Work out the finished part from the listing and answer in its coordinate system (mm). Coordinates: 2 decimals unless noted, no trailing zeros. One line per item, written item: value.
```python
from build123d import *

# Parameters (mm, degrees)
SZKIC1_R                    = 3.4
DODANIE_WYCI_GNI_CIE1_DEPTH = 820


with BuildPart() as part:
    # Szkic1 → Dodanie-wyciągnięcie1 (new body)
    with BuildSketch(Plane.XY):
        with BuildLine():
            Line((-40, -19), (-40, 19))
            ThreePointArc((-40, 19), (-39.707106781, 19.707106781), (-39, 20))
            Line((-39, 20), (-24, 20))
            Line((-24, 20), (-24, 15.5))
            Line((-24, 15.5), (-26.471381771, 15.5))
            Line((-26.471381771, 15.5), (-26.471381771, 17.75))
            ThreePointArc((-26.471381771, 17.75), (-28.062372029, 17.090990258), (-28.721381771, 15.5))
            ThreePointArc((-28.721381771, 15.5), (-27.448087912, 10.962546258), (-24, 7.75))
            Line((-24, 7.75), (-16, 7.75))
            ThreePointArc((-16, 7.75), (-12.551912088, 10.962546258), (-11.278618229, 15.5))
            ThreePointArc((-11.278618229, 15.5), (-11.937627971, 17.090990258), (-13.528618229, 17.75))
            Line((-13.528618229, 17.75), (-13.528618229, 15.5))
            Line((-13.528618229, 15.5), (-16, 15.5))
            Line((-16, 15.5), (-16, 20))
            Line((-16, 20), (13.528618229, 20))
            Line((13.528618229, 20), (16, 20))
            Line((16, 20), (16, 15.5))
            Line((16, 15.5), (13.528618229, 15.5))
            Line((13.528618229, 15.5), (13.528618229, 17.75))
            ThreePointArc((13.528618229, 17.75), (11.937627971, 17.090990258), (11.278618229, 15.5))
            ThreePointArc((11.278618229, 15.5), (12.551912088, 10.962546258), (16, 7.75))
            Line((16, 7.75), (24, 7.75))
            ThreePointArc((24, 7.75), (27.448087912, 10.962546258), (28.721381771, 15.5))
            ThreePointArc((28.721381771, 15.5), (28.062372029, 17.090990258), (26.471381771, 17.75))
            Line((26.471381771, 17.75), (26.471381771, 15.5))
            Line((26.471381771, 15.5), (24, 15.5))
            Line((24, 15.5), (24, 20))
            Line((24, 20), (39, 20))
            ThreePointArc((39, 20), (39.707106781, 19.707106781), (40, 19))
            Line((40, 19), (40, 4))
            Line((40, 4), (35.5, 4))
            Line((35.5, 4), (35.5, 6.471381771))
            Line((35.5, 6.471381771), (37.75, 6.471381771))
            ThreePointArc((37.75, 6.471381771), (37.090990258, 8.062372029), (35.5, 8.721381771))
            ThreePointArc((35.5, 8.721381771), (30.962546258, 7.448087912), (27.75, 4))
            Line((27.75, 4), (27.75, -4))
            ThreePointArc((27.75, -4), (30.962546258, -7.448087912), (35.5, -8.721381771))
            ThreePointArc((35.5, -8.721381771), (37.090990258, -8.062372029), (37.75, -6.471381771))
            Line((37.75, -6.471381771), (35.5, -6.471381771))
            Line((35.5, -6.471381771), (35.5, -4))
            Line((35.5, -4), (40, -4))
            Line((40, -4), (40, -19))
            ThreePointArc((40, -19), (39.707106781, -19.707106781), (39, -20))
            Line((39, -20), (24, -20))
            Line((24, -20), (24, -15.5))
            Line((24, -15.5), (26.471381771, -15.5))
            Line((26.471381771, -15.5), (26.471381771, -17.75))
            ThreePointArc((26.471381771, -17.75), (28.062372029, -17.090990258), (28.721381771, -15.5))
            ThreePointArc((28.721381771, -15.5), (27.448087912, -10.962546258), (24, -7.75))
            Line((24, -7.75), (16, -7.75))
            ThreePointArc((16, -7.75), (12.551912088, -10.962546258), (11.278618229, -15.5))
            ThreePointArc((11.278618229, -15.5), (11.937627971, -17.090990258), (13.528618229, -17.75))
            Line((13.528618229, -17.75), (13.528618229, -15.5))
            Line((13.528618229, -15.5), (16, -15.5))
            Line((16, -15.5), (16, -20))
            Line((16, -20), (-16, -20))
            Line((-16, -20), (-16, -15.5))
            Line((-16, -15.5), (-13.528618229, -15.5))
            Line((-13.528618229, -15.5), (-13.528618229, -17.75))
            ThreePointArc((-13.528618229, -17.75), (-11.937627971, -17.090990258), (-11.278618229, -15.5))
            ThreePointArc((-11.278618229, -15.5), (-12.551912088, -10.962546258), (-16, -7.75))
            Line((-16, -7.75), (-24, -7.75))
            ThreePointArc((-24, -7.75), (-27.448087912, -10.962546258), (-28.721381771, -15.5))
            ThreePointArc((-28.721381771, -15.5), (-28.062372029, -17.090990258), (-26.471381771, -17.75))
            Line((-26.471381771, -17.75), (-26.471381771, -15.5))
            Line((-26.471381771, -15.5), (-24, -15.5))
            Line((-24, -15.5), (-24, -20))
            Line((-24, -20), (-39, -20))
            ThreePointArc((-39, -20), (-39.707106781, -19.707106781), (-40, -19))
        make_face()
        with Locations(Location((-20, 0, 0), (0, 0, 180))):
            Circle(SZKIC1_R, mode=Mode.SUBTRACT)
        with Locations(Location((20, 0, 0), (0, 0, 180))):
            Circle(SZKIC1_R, mode=Mode.SUBTRACT)
        with BuildLine():
            Line((30.971381771, -17.75), (36.75, -17.75))
            ThreePointArc((36.75, -17.75), (37.457106781, -17.457106781), (37.75, -16.75))
            Line((37.75, -16.75), (37.75, -10.971381771))
            Line((37.75, -10.971381771), (30.971381771, -10.971381771))
            Line((30.971381771, -10.971381771), (30.971381771, -17.75))
        make_face(mode=Mode.SUBTRACT)
        with BuildLine():
            Line((-35.5, -6.471381771), (-37.75, -6.471381771))
            ThreePointArc((-37.75, -6.471381771), (-37.090990258, -8.062372029), (-35.5, -8.721381771))
            ThreePointArc((-35.5, -8.721381771), (-30.962546258, -7.448087912), (-27.75, -4))
            Line((-27.75, -4), (-27.75, 4))
            ThreePointArc((-27.75, 4), (-30.962546258, 7.448087912), (-35.5, 8.721381771))
            ThreePointArc((-35.5, 8.721381771), (-37.090990258, 8.062372029), (-37.75, 6.471381771))
            Line((-37.75, 6.471381771), (-35.5, 6.471381771))
            Line((-35.5, 6.471381771), (-35.5, 4))
            Line((-35.5, 4), (-37.75, 4))
            Line((-37.75, 4), (-37.75, -4))
            Line((-37.75, -4), (-35.5, -4))
            Line((-35.5, -4), (-35.5, -6.471381771))
        make_face(mode=Mode.SUBTRACT)
        with BuildLine():
            Line((10.528618229, 7.090188806), (11.40950808, 7.090188806))
            ThreePointArc((11.40950808, 7.090188806), (12.470168251, 6.650848977), (12.90950808, 5.590188806))
            Line((12.90950808, 5.590188806), (12.90950808, -5.590188806))
            ThreePointArc((12.90950808, -5.590188806), (12.470168251, -6.650848977), (11.40950808, -7.090188806))
            Line((11.40950808, -7.090188806), (10.528618229, -7.090188806))
            ThreePointArc((10.528618229, -7.090188806), (9.467958057, -7.529528634), (9.028618229, -8.590188806))
            Line((9.028618229, -8.590188806), (9.028618229, -16.25))
            ThreePointArc((9.028618229, -16.25), (8.589278401, -17.310660172), (7.528618229, -17.75))
            Line((7.528618229, -17.75), (-7.528618229, -17.75))
            ThreePointArc((-7.528618229, -17.75), (-8.589278401, -17.310660172), (-9.028618229, -16.25))
            Line((-9.028618229, -16.25), (-9.028618229, -8.590188806))
            ThreePointArc((-9.028618229, -8.590188806), (-9.467958057, -7.529528634), (-10.528618229, -7.090188806))
            Line((-10.528618229, -7.090188806), (-11.40950808, -7.090188806))
            ThreePointArc((-11.40950808, -7.090188806), (-12.470168251, -6.650848977), (-12.90950808, -5.590188806))
            Line((-12.90950808, -5.590188806), (-12.90950808, 5.590188806))
            ThreePointArc((-12.90950808, 5.590188806), (-12.470168251, 6.650848977), (-11.40950808, 7.090188806))
            Line((-11.40950808, 7.090188806), (-10.528618229, 7.090188806))
            ThreePointArc((-10.528618229, 7.090188806), (-9.467958057, 7.529528634), (-9.028618229, 8.590188806))
            Line((-9.028618229, 8.590188806), (-9.028618229, 16.25))
            ThreePointArc((-9.028618229, 16.25), (-8.589278401, 17.310660172), (-7.528618229, 17.75))
            Line((-7.528618229, 17.75), (7.528618229, 17.75))
            ThreePointArc((7.528618229, 17.75), (8.589278401, 17.310660172), (9.028618229, 16.25))
            Line((9.028618229, 16.25), (9.028618229, 8.590188806))
            ThreePointArc((9.028618229, 8.590188806), (9.467958057, 7.529528634), (10.528618229, 7.090188806))
        make_face(mode=Mode.SUBTRACT)
        with BuildLine():
            Line((30.971381771, 10.971381771), (37.75, 10.971381771))
            Line((37.75, 10.971381771), (37.75, 16.75))
            ThreePointArc((37.75, 16.75), (37.457106781, 17.457106781), (36.75, 17.75))
            Line((36.75, 17.75), (30.971381771, 17.75))
            Line((30.971381771, 17.75), (30.971381771, 10.971381771))
        make_face(mode=Mode.SUBTRACT)
        with BuildLine():
            Line((-30.971381771, -10.971381771), (-30.971381771, -17.75))
            Line((-30.971381771, -17.75), (-36.75, -17.75))
            ThreePointArc((-36.75, -17.75), (-37.457106781, -17.457106781), (-37.75, -16.75))
            Line((-37.75, -16.75), (-37.75, -10.971381771))
            Line((-37.75, -10.971381771), (-30.971381771, -10.971381771))
        make_face(mode=Mode.SUBTRACT)
        with BuildLine():
            Line((-30.971381771, 17.75), (-36.75, 17.75))
            ThreePointArc((-36.75, 17.75), (-37.457106781, 17.457106781), (-37.75, 16.75))
            Line((-37.75, 16.75), (-37.75, 10.971381771))
            Line((-37.75, 10.971381771), (-30.971381771, 10.971381771))
            Line((-30.971381771, 10.971381771), (-30.971381771, 17.75))
        make_face(mode=Mode.SUBTRACT)
    extrude(amount=DODANIE_WYCI_GNI_CIE1_DEPTH)


solid = part.part
```
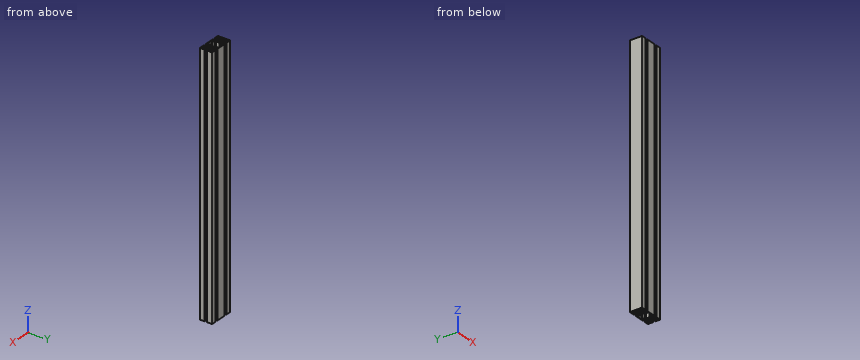
Item 1: Section A-A, the plane z = 377 is taken. Give the number of separate pieces and of enclosed holes in the cut face, then the cut area to 3 significant figures.
Evaluation:
separate pieces: 1
enclosed holes: 8
area: 1,260 mm2
Item 2: Consider probe 1 along X at (y, z) = (-15, 313); probe 2 along Y at (x, z) = (14.5, 518); probe 3 along Y at (x, z) = (34.5, 571). Determine where each line is inside the solid, lowest interval first.
Evaluation:
probe 1: x = -40 to -37.75, -30.97 to -28.71, -11.29 to -9.03, 9.03 to 11.29, 28.71 to 30.97, 37.75 to 40
probe 2: y = -20 to -15.5, -8.73 to 8.73, 15.5 to 20
probe 3: y = -20 to -17.75, -10.97 to -8.66, 8.66 to 10.97, 17.75 to 20
Item 3: Given pin 1 (4 mm diameter, centred on x = 19.5, z = 462, fed in from -Y), flat-ended and moving along its own axis, determine where the tip first touches the part or whether it passes through.
Evaluation:
pin 1: stops at y = -7.75
